Check sheet for the modelled part. Datum: model origin and axes. Units: mm. Give positions to 0.01 mm unless a question says otherwise; leave off trailing zeros. Write each loop counter-clockwise with the first axis right and the second up, starting at its lowest first coordinate (ties: lowest second). Pieces come first, ordered by that corner, then holes. Notation, with made-up numbers: (13, 17) -> (21, 17) arc R16 ccw to (21, 37) -> close; hole circle Ø6 at (-4.75, 31). An arc over 180 degrees is marked (long way). Answer as a JSON object with one key per item and string values.
from build123d import *

# Parameters (mm, degrees)
F1_DEPTH = 0.1


with BuildPart() as f1:
    # F0 (on Front) → F1 (new body)
    with BuildSketch(Plane.XZ):
        with BuildLine():
            ThreePointArc((4.8052448645, 4.2392099088), (5.9938653468, 2.2660223), (6.4079075258, 0))
            ThreePointArc((6.4079075258, 0), (5.9938653468, -2.2660223), (4.8052448645, -4.2392099088))
            ThreePointArc((4.8052448645, -4.2392099088), (6.8764974545, -5.5075560727), (8.4202976896, -7.38251477))
            ThreePointArc((8.4202976896, -7.38251477), (19.6961982172, 0.7329368237), (7.1375086194, 6.6731222471))
            ThreePointArc((7.1375086194, 6.6731222471), (6.0935080211, 5.3391354228), (4.8052448645, 4.2392099088))
        make_face()
        with BuildLine():
            ThreePointArc((7.1375086194, 6.6731222471), (5.8427804889, 5.5793917075), (4.8052448645, 4.2392099088))
            ThreePointArc((4.8052448645, 4.2392099088), (6.0935080211, 5.3391354228), (7.1375086194, 6.6731222471))
        make_face()
        with BuildLine():
            ThreePointArc((-4.8283466328, 4.2128787845), (-0.0175144213, 6.4078835901), (4.8052448645, 4.2392099088))
            ThreePointArc((4.8052448645, 4.2392099088), (5.8427804889, 5.5793917075), (7.1375086194, 6.6731222471))
            ThreePointArc((7.1375086194, 6.6731222471), (-1.5477052479, 19.5526553507), (-5.1442647229, 4.4404062517))
            ThreePointArc((-5.1442647229, 4.4404062517), (-4.9848340595, 4.3286858356), (-4.8283466328, 4.2128787845))
        make_face()
        with BuildLine():
            ThreePointArc((8.4202976896, -7.38251477), (6.3739752542, -6.0854969279), (4.8052448645, -4.2392099088))
            ThreePointArc((4.8052448645, -4.2392099088), (1.1757337965, -6.2991212799), (-2.9524774752, -5.6871922438))
            ThreePointArc((-2.9524774752, -5.6871922438), (-3.534399564, -6.5137001688), (-4.2218378667, -7.2547651103))
            ThreePointArc((-4.2218378667, -7.2547651103), (1.9874253454, -18.3828453768), (8.4202976896, -7.38251477))
        make_face()
        with BuildLine():
            ThreePointArc((8.4202976896, -7.38251477), (6.8764974545, -5.5075560727), (4.8052448645, -4.2392099088))
            ThreePointArc((4.8052448645, -4.2392099088), (6.3739752542, -6.0854969279), (8.4202976896, -7.38251477))
        make_face()
        with BuildLine():
            ThreePointArc((-2.9524774752, -5.6871922438), (-6.2958841747, -1.1929464859), (-4.8283466328, 4.2128787845))
            ThreePointArc((-4.8283466328, 4.2128787845), (-4.9876113011, 4.324829682), (-5.1442647229, 4.4404062517))
            ThreePointArc((-5.1442647229, 4.4404062517), (-16.8849803616, -2.3695755088), (-4.2218378667, -7.2547651103))
            ThreePointArc((-4.2218378667, -7.2547651103), (-3.6412753486, -6.427156257), (-2.9524774752, -5.6871922438))
        make_face()
        with BuildLine():
            ThreePointArc((-5.1442647229, 4.4404062517), (-4.9876113011, 4.324829682), (-4.8283466328, 4.2128787845))
            ThreePointArc((-4.8283466328, 4.2128787845), (-4.9848340595, 4.3286858356), (-5.1442647229, 4.4404062517))
        make_face()
        with BuildLine():
            ThreePointArc((-4.2218378667, -7.2547651103), (-3.534399564, -6.5137001688), (-2.9524774752, -5.6871922438))
            ThreePointArc((-2.9524774752, -5.6871922438), (-3.6412753486, -6.427156257), (-4.2218378667, -7.2547651103))
        make_face()
    extrude(amount=F1_DEPTH)


solid = f1.part
1. Sectioned sample at A-A, the plane z = -2. Enter the section's corners in (x, y) (3 decimals), plus the area to 3 significant figures.
Determined:
{"outline": "(-16.905, -0.1) -> (-6.088, -0.1) -> (-6.088, 0) -> (-16.905, 0) -> close; (6.088, -0.1) -> (19.478, -0.1) -> (19.478, 0) -> (6.088, 0) -> close", "area": "2.42 mm^2"}
2. Sectioned sample at B-B, the plane x = -2.5. Enter the section's corners in (y, z), plus the area to 3 significant figures.
Determined:
{"outline": "(-0.1, -16.79) -> (0, -16.79) -> (0, -5.9) -> (-0.1, -5.9) -> close; (-0.1, 5.9) -> (0, 5.9) -> (0, 19.32) -> (-0.1, 19.32) -> close", "area": "2.43 mm^2"}
3. Sectioned sample at C-C, the plane y = -0.05. Enter the section's corners in (x, z).
Determined:
{"outline": "(-5.14, 4.44) arc R7.53 ccw (long way) to (-4.22, -7.25) arc R7.34 ccw (long way) to (8.42, -7.38) arc R8.06 ccw (long way) to (7.14, 6.67) arc R8.48 ccw (long way) to start; hole circle Ø12.82 at (0, 0)"}
4. Scan line: L1, parallel to Z at x = 11, y = -0.05. Record every from-to range of solid material in increasing order. Write a range as [from, to].
Determined:
{"L1": "[-8.04, 8.04]"}
5. Sectioned sample at D-D, the plane z = 5. Enter the section's corners in (x, y).
Determined:
{"outline": "(-12.65, -0.1) -> (-6.11, -0.1) -> (-6.11, 0) -> (-12.65, 0) -> close; (-5.81, -0.1) -> (-4.01, -0.1) -> (-4.01, 0) -> (-5.81, 0) -> close; (4.01, -0.1) -> (17.99, -0.1) -> (17.99, 0) -> (4.01, 0) -> close"}
